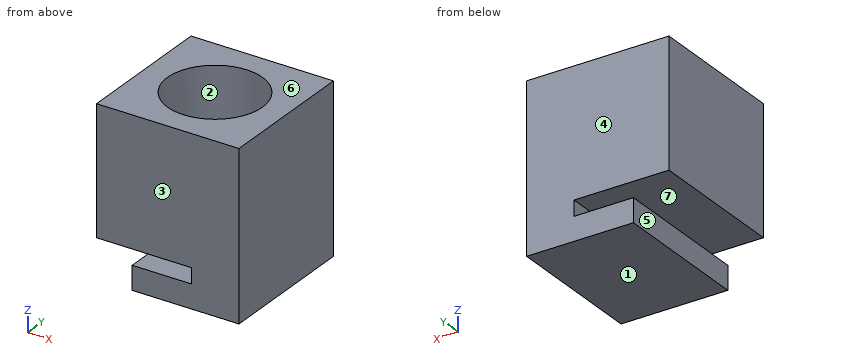
```python
from build123d import *

# Parameters (mm, degrees)
ESQUISSE1_W             = 12
ESQUISSE1_H             = 12
BOSS_EXTRU_1_DEPTH      = 14
ESQUISSE2_R             = 4
ENL_V_MAT_EXTRU_1_DEPTH = 6
ESQUISSE3_W             = 1.3
ESQUISSE3_H             = 14.296544168
ENL_V_MAT_EXTRU_2_DEPTH = 18
ESQUISSE6_W             = 2.656896507
ESQUISSE6_H             = 12.791812985
ENL_V_MAT_EXTRU_4_DEPTH = 13


with BuildPart() as part:
    # Esquisse1 → Boss.-Extru.1 (new body)
    with BuildSketch(Plane.XY):
        Rectangle(ESQUISSE1_W, ESQUISSE1_H)
    extrude(amount=BOSS_EXTRU_1_DEPTH)

    # Esquisse2 → Enlèv. mat.-Extru.1 (cut)
    with BuildSketch(Plane.XY.offset(14)):
        Circle(ESQUISSE2_R)
    extrude(amount=-ENL_V_MAT_EXTRU_1_DEPTH, mode=Mode.SUBTRACT)

    # Esquisse3 → Enlèv. mat.-Extru.2 (cut)
    with BuildSketch(Plane.ZY.offset(16)):
        with Locations((2.65, 0)):
            Rectangle(ESQUISSE3_W, ESQUISSE3_H)
    extrude(amount=-ENL_V_MAT_EXTRU_2_DEPTH, mode=Mode.SUBTRACT)

    # Esquisse6 → Enlèv. mat.-Extru.4 (cut)
    with BuildSketch(Plane.ZY.offset(16)):
        with Locations((0.90678419, -0.070381364)):
            Rectangle(ESQUISSE6_W, ESQUISSE6_H)
    extrude(amount=-ENL_V_MAT_EXTRU_4_DEPTH, mode=Mode.SUBTRACT)


solid = part.part
```
Can you work these out from the model? Positions are in its coordinate system, mm. Face numbers are marked on the shaded views. A direction names the side the tool comes from. Round coordinates to 2 decimals unless told otherwise and drop trailing zeros. Loops run counter-clockwise (first coordinate to the right, second up) from the corner with the lowest first, then second, coordinate; pieces in that order, holes last. Notation, with made-up numbers: M -1.75,-23 L 23.25,-23 A6 cw 23.25,-17 Z; hole C 63.25,69 d6. An arc over 180 degrees is marked long. Answer as a JSON object with one key per item and string values. Group by question number.
Q1. We'd pull the mould along Y, two halves only. Please class the marked faces 1, 2, 3 and 4: +Y half, -Y half, draft (parallel to the pull), parting line (faces both ways), or undercut.
Q2. Imagine slicing it at A-A, the plane x = 0. Please give me the cut outline in (y, z).
Q3. Will these pins go through, and if not, where does the flat tip stop? pin 1 (2.5 mm diameter, centred on x = 0, y = 1.5, fed in from +Z); pin 2 (1.6 mm diameter, centred on y = 0.5, z = 0.5, fed in from -X).
Q4. On a 3-axis mill with a long thin cutter (end or side, diameter ignored), from which of +Z, -Z, +X, -X, +Y, -Y can I reach the whole of each face in a straight line? I mean the marked faces 5, 6 and 7. Say none if no direction works.
Q5. Imagine slicing it at B-B, the plane z = 12.25. Please give me the cut outline in (x, y), then the cut area to 3 significant figures.
Q6. Please list where these lines run through material, in increasing order: L1, parallel to Y at x = 0, z = 11.85; L2, parallel to Z at x = -1.75, y = 1; L3, parallel to Z at x = 1.5, y = 5.25.
Q7. Imagine slicing it at D-D, the plane y = -5. Please give me the cut outline in (x, z), then the cut area to 3 significant figures.
Q8. Imagine slicing it at C-C, the plane y = 0. Please give me the cut outline in (x, z), then the cut area to 3 significant figures.
Findings:
{
 "1": {"face 1": "draft", "face 2": "undercut", "face 3": "-Y half", "face 4": "+Y half"},
 "2": {"outline": "M -6,0 L 6,0 L 6,2 L -6,2 Z; M -6,3.3 L 6,3.3 L 6,14 L 4,14 L 4,8 L -4,8 L -4,14 L -6,14 Z"},
 "3": {"pin 1": "stops at z = 8", "pin 2": "stops at x = -3"},
 "4": {"face 5": "-Z, -X, +Y, -Y", "face 6": "+Z, +X, -X, +Y, -Y", "face 7": "-X, +Y, -Y"},
 "5": {"outline": "M -6,-6 L 6,-6 L 6,6 L -6,6 Z; hole C 0,0 d8", "area": "93.7 mm2"},
 "6": {"L1": "y = -6 to -4, 4 to 6", "L2": "z = 0 to 2, 3.3 to 8", "L3": "z = 0 to 2, 3.3 to 14"},
 "7": {"outline": "M -6,3.3 L 2,3.3 L 2,2 L -3,2 L -3,0 L 6,0 L 6,14 L -6,14 Z", "area": "152 mm2"},
 "8": {"outline": "M -6,3.3 L 2,3.3 L 2,2 L -3,2 L -3,0 L 6,0 L 6,14 L 4,14 L 4,8 L -4,8 L -4,14 L -6,14 Z", "area": "104 mm2"}
}
